from build123d import *

# Parameters (mm, degrees)
BOSS_EXTRUDE1_DEPTH = 3
SKETCH2_W           = 65
SKETCH2_H           = 3
BOSS_EXTRUDE2_DEPTH = 65
CUT_EXTRUDE1_REACH  = 114.663
SKETCH3_R           = 2.5
SKETCH3_R_2         = 19.1
SKETCH4_R           = 19.1
SKETCH4_R_2         = 2.5
BOSS_EXTRUDE3_DEPTH = 3
SKETCH5_W           = 65
SKETCH5_H           = 66.483873972
CUT_EXTRUDE2_DEPTH  = 3
SKETCH6_R           = 2.5
CUT_EXTRUDE3_DEPTH  = 3
BOSS_EXTRUDE5_DEPTH = 3
BOSS_EXTRUDE6_DEPTH = 3


with BuildPart() as part:
    # Sketch1 → Boss-Extrude1 (new body)
    with BuildSketch(Plane(origin=(0, 0, 0), x_dir=(1, 0, 0), z_dir=(0, 1, 0))):
        Polygon((52.5, 0), (59, 0), (65, 6), (65, 65), (0, 65), (0, 6), (6, 0), align=None)
        with BuildLine():
            ThreePointArc((54.6, 10), (53.98492424, 8.51507576), (52.5, 7.9))
            ThreePointArc((52.5, 7.9), (51.01507576, 8.51507576), (50.4, 10))
            Line((50.4, 10), (50.4, 52))
            ThreePointArc((50.4, 52), (52.5, 54.1), (54.6, 52))
            Line((54.6, 52), (54.6, 10))
        make_face(mode=Mode.SUBTRACT)
        with BuildLine():
            Line((14.6, 52), (14.624057294, 52))
            Line((14.624057294, 52), (14.6, 10))
            ThreePointArc((14.6, 10), (12.5, 7.9), (10.4, 10))
            Line((10.4, 10), (10.4, 52))
            ThreePointArc((10.4, 52), (12.5, 54.1), (14.6, 52))
        make_face(mode=Mode.SUBTRACT)
    extrude(amount=BOSS_EXTRUDE1_DEPTH)

    # Sketch2 → Boss-Extrude2 (add)
    with BuildSketch(Plane(origin=(0, 3, 0), x_dir=(1, 0, 0), z_dir=(0, 1, 0))):
        with Locations((32.5, 63.5)):
            Rectangle(SKETCH2_W, SKETCH2_H)
    extrude(amount=BOSS_EXTRUDE2_DEPTH)

    # Sketch3 → Cut-Extrude1 (cut, up to next)
    with BuildSketch(Plane.XY.offset(-62), mode=Mode.PRIVATE) as cut_extrude1_sk1:
        Polygon((6, 68), (0, 68), (0, 62), align=None)
    cut_extrude1_tool1 = extrude(cut_extrude1_sk1.sketch, amount=-CUT_EXTRUDE1_REACH, mode=Mode.PRIVATE) & part.part
    # Sketch3 → Cut-Extrude1 (cut, up to next)
    with BuildSketch(Plane.XY.offset(-62), mode=Mode.PRIVATE) as cut_extrude1_sk2:
        with Locations((8.93, 15.43)):
            Circle(SKETCH3_R)
    cut_extrude1_tool2 = extrude(cut_extrude1_sk2.sketch, amount=-CUT_EXTRUDE1_REACH, mode=Mode.PRIVATE) & part.part
    # Sketch3 → Cut-Extrude1 (cut, up to next)
    with BuildSketch(Plane.XY.offset(-62), mode=Mode.PRIVATE) as cut_extrude1_sk3:
        with Locations((56.07, 15.43)):
            Circle(SKETCH3_R)
    cut_extrude1_tool3 = extrude(cut_extrude1_sk3.sketch, amount=-CUT_EXTRUDE1_REACH, mode=Mode.PRIVATE) & part.part
    # Sketch3 → Cut-Extrude1 (cut, up to next)
    with BuildSketch(Plane.XY.offset(-62), mode=Mode.PRIVATE) as cut_extrude1_sk4:
        with Locations((56.07, 62.57)):
            Circle(SKETCH3_R)
    cut_extrude1_tool4 = extrude(cut_extrude1_sk4.sketch, amount=-CUT_EXTRUDE1_REACH, mode=Mode.PRIVATE) & part.part
    # Sketch3 → Cut-Extrude1 (cut, up to next)
    with BuildSketch(Plane.XY.offset(-62), mode=Mode.PRIVATE) as cut_extrude1_sk5:
        with Locations((32.5, 39)):
            Circle(SKETCH3_R_2)
    cut_extrude1_tool5 = extrude(cut_extrude1_sk5.sketch, amount=-CUT_EXTRUDE1_REACH, mode=Mode.PRIVATE) & part.part
    # Sketch3 → Cut-Extrude1 (cut, up to next)
    with BuildSketch(Plane.XY.offset(-62), mode=Mode.PRIVATE) as cut_extrude1_sk6:
        Polygon((65, 68), (59, 68), (65, 62), align=None)
    cut_extrude1_tool6 = extrude(cut_extrude1_sk6.sketch, amount=-CUT_EXTRUDE1_REACH, mode=Mode.PRIVATE) & part.part
    # Sketch3 → Cut-Extrude1 (cut, up to next)
    with BuildSketch(Plane.XY.offset(-62), mode=Mode.PRIVATE) as cut_extrude1_sk7:
        with BuildLine():
            ThreePointArc((11.43, 62.57), (7.214795913, 64.388811408), (8.783540049, 60.074293791))
            ThreePointArc((8.783540049, 60.074293791), (10.645204087, 60.751188592), (11.43, 62.57))
        make_face()
    cut_extrude1_tool7 = extrude(cut_extrude1_sk7.sketch, amount=-CUT_EXTRUDE1_REACH, mode=Mode.PRIVATE) & part.part
    add(cut_extrude1_tool1.solids().sort_by_distance((2, 66, -62))[0], mode=Mode.SUBTRACT)
    add(cut_extrude1_tool2.solids().sort_by_distance((8.93, 15.43, -62))[0], mode=Mode.SUBTRACT)
    add(cut_extrude1_tool3.solids().sort_by_distance((56.07, 15.43, -62))[0], mode=Mode.SUBTRACT)
    add(cut_extrude1_tool4.solids().sort_by_distance((56.07, 62.57, -62))[0], mode=Mode.SUBTRACT)
    add(cut_extrude1_tool5.solids().sort_by_distance((32.5, 39, -62))[0], mode=Mode.SUBTRACT)
    add(cut_extrude1_tool6.solids().sort_by_distance((63, 66, -62))[0], mode=Mode.SUBTRACT)
    add(cut_extrude1_tool7.solids().sort_by_distance((8.93, 62.57, -62))[0], mode=Mode.SUBTRACT)

    # Sketch4 → Boss-Extrude3 (add)
    with BuildSketch(Plane(origin=(0, 0, -65), x_dir=(-1, 0, 0), z_dir=(0, 0, -1))):
        Polygon((-65, 62), (-59, 68), (-6, 68), (0, 62), (0, 0), (-65, 0), align=None)
        with Locations(Location((-32.5, 39, 0), (0, 0, 180))):
            Circle(SKETCH4_R, mode=Mode.SUBTRACT)
        with Locations(Location((-56.07, 62.57, 0), (0, 0, 180))):
            Circle(SKETCH4_R_2, mode=Mode.SUBTRACT)
        with Locations(Location((-8.93, 62.57, 0), (0, 0, 180))):
            Circle(SKETCH4_R_2, mode=Mode.SUBTRACT)
    extrude(amount=BOSS_EXTRUDE3_DEPTH)

    # Sketch5 → Cut-Extrude2 (cut)
    with BuildSketch(Plane.XY.offset(-62)):
        with Locations((32.5, 36.241936986)):
            Rectangle(SKETCH5_W, SKETCH5_H)
    extrude(amount=-CUT_EXTRUDE2_DEPTH, mode=Mode.SUBTRACT)

    # Sketch6 → Cut-Extrude3 (cut)
    with BuildSketch(Plane(origin=(0, 0, -68), x_dir=(-1, 0, 0), z_dir=(0, 0, -1))):
        with Locations((-56.07, 15.43)):
            Circle(SKETCH6_R)
        with Locations((-8.93, 15.43)):
            Circle(SKETCH6_R)
    extrude(amount=-CUT_EXTRUDE3_DEPTH, mode=Mode.SUBTRACT)

    # Sketch7 → Boss-Extrude5 (add)
    with BuildSketch(Plane.ZY):
        Polygon((-65, 3), (-50, 3), (-65, 28), align=None)
    extrude(amount=-BOSS_EXTRUDE5_DEPTH)

    # Sketch8 → Boss-Extrude6 (add)
    with BuildSketch(Plane(origin=(65, 0, 0), x_dir=(0, 0, -1), z_dir=(1, 0, 0))):
        Polygon((65, 3), (50, 3), (65, 28), align=None)
    extrude(amount=-BOSS_EXTRUDE6_DEPTH)


solid = part.part
Source: CAD feature listing. Evaluate the final solid. Frame: model axes, mm. A direction names the side the tool comes from. Give positions to 0.01 mm unless a question says otherwise; leave off trailing zeros. Write each loop counter-clockwise with the first axis right and the second up, starting at its lowest first coordinate (ties: lowest second). Pieces come first, ordered by that corner, then holes. Notation, with made-up numbers: M 84.5,14 L 139.5,14 A18 ccw 139.5,33 Z; hole C -40,-2.5 d5. An arc over 180 degrees is marked long. Return JSON: item names as keys, results as strings. Group by question number.
1) First-contact query: pin 1 Ø4 at (x, y) = (8.93, 62.57) entering from -Z; pin 2 Ø1.5 at (x, z) = (24.5, -18.5) entering from +Y; pin 3 Ø1.5 at (x, y) = (43.5, 11) entering from +Z. Flat tips, straight axial feed; report the tip coordinate or a pass-through.
2) Draft query along X for faces 4 (the face through (62, 1, -3)), 5 (the face through (41.313, 55.945, -66.479)), 6 (the face through (63.521, 15.325, -57.395)). Return one class per face: released by +X, released by -X, zero draft, split by the parting line, or undercut.
3) Set-up query: faces 1 (the face through (62, 65, -66)), 2 (the face through (52.5, 1.5, -54.1)), 3 (the face through (46, 22, -65)). Return all of +Z, -Z, +X, -X, +Y, -Y with unobstructed straight access to the full face (end or side cutting, diameter ignored); none if empty.
4) Cut plane A-A, the plane x = 56.07. Output: boundary loops of the cut face in (y, z).
5) Cut plane D-D, the plane z = -62. Output: boundary loops of the cut face in (x, y), then the cut area to 3 significant figures.
6) Cut plane C-C, the plane x = 32.5. Output: boundary loops of the cut face in (y, z).
7) Ray query, L1, parallel to Y at x = 8.93, z = -66; L2, parallel to X at y = 62.57, z = -67; L3, parallel to X at y = 10.5, z = -58. Return the intervals inside material, ascending.
8) Cut plane B-B, the plane y = 39. Output: boundary loops of the cut face in (x, z), then the cut area to 3 significant figures.
Data:
{
 "1": {"pin 1": "passes through", "pin 2": "stops at y = 3", "pin 3": "stops at z = -65"},
 "2": {"face 4": "released by +X", "face 5": "undercut", "face 6": "zero draft"},
 "3": {"face 1": "+Z, -Z, +X, +Y", "face 2": "+Y, -Y", "face 3": "+Z, +Y"},
 "4": {"outline": "M 0,-68 L 12.93,-68 L 12.93,-65 L 3,-65 L 3,0 L 0,0 Z; M 17.93,-68 L 60.07,-68 L 60.07,-65 L 17.93,-65 Z; M 65.07,-68 L 68,-68 L 68,-65 L 65.07,-65 Z"},
 "5": {"outline": "M 0,0 L 65,0 L 65,23 L 62,23 L 62,3 L 3,3 L 3,23 L 0,23 Z", "area": "315 mm²"},
 "6": {"outline": "M 0,-68 L 19.9,-68 L 19.9,-65 L 3,-65 L 3,0 L 0,0 Z; M 58.1,-68 L 68,-68 L 68,-65 L 58.1,-65 Z"},
 "7": {"L1": "y = 0 to 12.93, 17.93 to 60.07, 65.07 to 68", "L2": "x = 0.57 to 6.43, 11.43 to 53.57, 58.57 to 64.43", "L3": "x = 0 to 3, 62 to 65"},
 "8": {"outline": "M 0,-68 L 13.4,-68 L 13.4,-65 L 0,-65 Z; M 51.6,-68 L 65,-68 L 65,-65 L 51.6,-65 Z", "area": "80.4 mm²"}
}
